Autodesk Inventor part; units mm, degrees
ref_plane "YZ Plane" through (0, 0, 0) normal (1, 0, 0) x (0, 1, 0)
ref_plane "XZ Plane" through (0, 0, 0) normal (0, 1, 0) x (-1, 0, 0)
ref_plane "XY Plane" through (0, 0, 0) normal (0, 0, 1) x (1, 0, 0)
sketch "スケッチ1" plane through (0, 0, 0) normal (0, 0, 1) x (1, 0, 0)
  line L0 (-20, -2.5) -> (20, -2.5)
  line L1 (20, -2.5) -> (20, 2.5)
  line L2 (-20, 2.5) -> (-20, -2.5)
  line L3 (-20, -2.5) -> (20, 2.5) construction
  line L4 (20, -2.5) -> (-20, 2.5) construction
  line L5 (-10, 2.5) -> (10, 2.5)
  line L6 (10, 2.5) -> (10, 52.5)
  line L7 (10, 52.5) -> (-10, 52.5)
  line L8 (-10, 52.5) -> (-10, 2.5)
  line L9 (-10, 2.5) -> (10, 52.5) construction
  line L10 (10, 2.5) -> (-10, 52.5) construction
  line L11 (20, 2.5) -> (10, 2.5)
  line L12 (-10, 2.5) -> (-20, 2.5)
  point P0 (0, 0)
  point P1 (0, 27.5)
  point P2 (0, 27.5)
  point P3 (0, 0)
  dimension "d0" = 20
  dimension "d1" = 50
  dimension "d2" = 5
  dimension "d3" = 10
extrude "押し出し1" add sketch "スケッチ1" along normal mid plane 210
sketch "スケッチ4" plane through (20, -2.5, 105) normal (1, 0, 0) x (0, 0, -1)
  line L0 (0, 7) -> (33.61, 55)
  line L1 (210, 55) -> (0, 55)
  line L2 (0, 5) -> (0, 55)
  line L3 (210, 5) -> (0, 5)
  line L4 (210, 55) -> (210, 5)
  line L5 (0, 0) -> (0, 5)
  point P0 (105, 2.5)
  dimension "d18" = 35
  dimension "d21" = 2
extrude "押し出し3" cut sketch "スケッチ4" against normal through all contours L2 L1 L0
sketch "スケッチ6" plane through (10, 2.5, -105) normal (1, 0, 0) x (0, 0, -1)
  circle A0 centre (-159, 42) radius 6
  line L0 (0, 0) -> (-210, 0)
  line L1 (-210, -5) -> (-210, 0)
  point P0 (-105, -2.5)
  dimension "d33" = 12
  dimension "d34" = 42
  dimension "d35" = 51
extrude "押し出し4" cut sketch "スケッチ6" against normal through all
properties part number "s_base2"
Geometry check sheet. Reference: the model listing, model coordinates, mm. A direction names the side the tool comes from. Give positions to 0.01 mm unless a question says otherwise; leave off trailing zeros. Write each loop counter-clockwise with the first axis right and the second up, starting at its lowest first coordinate (ties: lowest second). Pieces come first, ordered by that corner, then holes.
1) Gauge pin test, flat ends, axial feed: pin 1 (15.5 mm diameter, centred on y = 44.5, z = 54, fed in from +X); pin 2 (3 mm diameter, centred on x = -5, y = 32, fed in from +Z); pin 3 (5 mm diameter, centred on x = -16.5, z = 22, fed in from +Y). Record the tip position at first contact, or that the pin passes through.
2) Section check A-A, the plane z = 54. Record the boundary of the cut face in (x, y).
3) Section check C-C, the plane z = 1.5. Record the boundary of the cut face in (x, y), and give its area (3 significant figures).
4) Release check for a two-part mould opening along Y. For faces 4 (the flat face through (10, 27, -1)), 5 (the flat face through (0, -2.5, -1)), 6 (the cylindrical face through (0.14, 44.764, 59.994)) record: pulls with the +Y half, pulls with the -Y half, needs draft (parallel to the pull), parting line crosses it, or undercut.
5) Material ranges on L1, parallel to Y at x = -1, z = 54; L2, parallel to Y at x = -15.5, z = -77; L3, parallel to X at y = 33, z = 21.5, recorded low to high.
6) Access from +Z, -Z, +X, -X, +Y, -Y to the whole of each face (thin tool, end or side, straight path). Record for faces 1 (the flat face through (0, 52.5, -18)), 2 (the flat face through (15, 2.5, -1)), 3 (the flat face through (-10, 28, -1)).
7) Section check B-B, the plane y = 44.5. Record the boundary of the cut face in (x, z).
8) Section check D-D, the plane x = 2. Record the boundary of the cut face in (y, z).
Computed:
1. pin 1: stops at x = 10
1. pin 2: stops at z = 86.79
1. pin 3: stops at y = 2.5
2. outline: (-20, -2.5) - (20, -2.5) - (20, 2.5) - (10, 2.5) - (10, 38.5) - (-10, 38.5) - (-10, 2.5) - (-20, 2.5) - close; (-10, 50.5) - (10, 50.5) - (10, 52.5) - (-10, 52.5) - close
3. outline: (-20, -2.5) - (20, -2.5) - (20, 2.5) - (10, 2.5) - (10, 52.5) - (-10, 52.5) - (-10, 2.5) - (-20, 2.5) - close
3. area: 1,200 mm2
4. face 4: needs draft
4. face 5: pulls with the -Y half
4. face 6: undercut
5. L1: y = -2.5 to 38.5, 50.5 to 52.5
5. L2: y = -2.5 to 2.5
5. L3: x = -10 to 10
6. face 1: +Z, -Z, +X, -X, +Y
6. face 2: +Z, -Z, +X, +Y
6. face 3: +Z, -Z, -X, +Y
7. outline: (-10, -105) - (10, -105) - (10, 48) - (-10, 48) - close; (-10, 60) - (10, 60) - (10, 76.99) - (-10, 76.99) - close
8. outline: (-2.5, -105) - (52.5, -105) - (52.5, 71.39) - (4.5, 105) - (-2.5, 105) - close; hole circle Ø12 at (44.5, 54)
